Build history of the part. All positions in model axes, mm. A direction names the side the tool comes from. Round coordinates to 2 decimals unless told otherwise and drop trailing zeros. Loops run counter-clockwise (first coordinate to the right, second up) from the corner with the lowest first, then second, coordinate; pieces in that order, holes last.
Autodesk Inventor part; units mm, degrees
ref_plane "YZ Plane" through (0, 0, 0) normal (1, 0, 0) x (0, 1, 0)
ref_plane "XZ Plane" through (0, 0, 0) normal (0, 1, 0) x (-1, 0, 0)
ref_plane "XY Plane" through (0, 0, 0) normal (0, 0, 1) x (1, 0, 0)
sketch "スケッチ1" plane through (0, 0, 0) normal (0, 0, 1) x (1, 0, 0)
  line L0 (0, -3.25) -> (0.8, -3.25)
  line L1 (0.8, -3.25) -> (1.1, -2.95)
  line L2 (1.1, -2.95) -> (1.1, 1.25)
  line L3 (1.1, 1.25) -> (1.1, 1.25)
  line L4 (1.1, 1.25) -> (1.1, 1.75)
  line L5 (1.1, 1.75) -> (2.2, 1.75)
  line L6 (2.5, 5.45) -> (2.2, 5.75)
  line L7 (2.2, 5.75) -> (1.5, 5.75)
  line L8 (1.5, 5.75) -> (1.2, 5.45)
  line L9 (0, 7.4044) -> (0, -7.4044) construction
  line L10 (0, -3.25) -> (0, 3.25)
  line L11 (0, 3.25) -> (1.2, 3.25)
  line L12 (1.2, 3.25) -> (1.2, 5.45)
  line L13 (2.2, 1.75) -> (2.5, 2.05)
  line L14 (2.5, 2.05) -> (2.5, 5.45)
  point P0 (0, 0)
  point P1 (0, 0)
  dimension "d0" = 2.2
  dimension "d1" = 5
  dimension "d2" = 0.3
  dimension "d3" = 0.3
  dimension "d4" = 2.2
  dimension "d5" = 0.5
  dimension "d6" = 4
  dimension "d8" = 0.3
  dimension "d9" = 2.4
  dimension "d10" = 2.5
  dimension "d11" = 0.3
  dimension "d12" = 0.3
  dimension "d13" = 0.3
  dimension "d14" = 0.3
  dimension "d15" = 5
revolve "回転1" add sketch "スケッチ1" angle 360 about axis through (0, 7.4044, 0) along (0, -1, 0)
sketch "スケッチ2" plane through (0, -3.25, 0) normal (0, -1, 0) x (1, 0, 0)
  circle A0 centre (0, 0) radius 0.8
  circle A1 centre (0, 0) radius 9.0242
extrude "押し出し1" cut sketch "スケッチ2" against normal blind 0.5 contours A0 | A1
sketch "スケッチ3" plane through (0, 5.75, 0) normal (0, 1, 0) x (1, 0, 0)
  circle A0 centre (0, 0) radius 2.5
  line L0 (2.5, 0) -> (-2.5, 0)
  line L1 (2.5, -0.5) -> (-2.5, -0.5)
  line L2 (2.5, 0.5) -> (-2.5, 0.5)
  line L3 (2.5, -0.5) -> (2.5, 0.5)
  line L4 (-2.5, -0.5) -> (-2.5, 0.5)
  point P0 (0, 0)
  point P1 (-2.4495, -0.5)
  point P2 (2.4495, -0.5)
  point P3 (2.4495, 0.5)
  point P4 (-2.4495, 0.5)
  dimension "d19" = 0.5
extrude "押し出し2" cut sketch "スケッチ3" against normal blind 1 contours L0 A0 L2 | A0 L1 L0
equation "\"d3\" = d2"
equation "\"d11\" = d8"
equation "\"d12\" = d8"
equation "\"d13\" = d12"
equation "\"d14\" = d13"
properties part number "BRU-2604S" material "ステンレス鋼 AISI 304"
(1) Pull direction X, two halves, no side cores. Call faces 6 (the face through (1.05, -0.47, -0.33)), 7 (the face through (-0.02, 5.57, 1.32)), 8 (the face through (2, 5, -0.5)): +X half, -X half, draft (parallel to the pull), parting line (faces both ways), or undercut.
Responses:
face 6: parting line
face 7: undercut
face 8: draft
(2) Slice it at B-B on x = 0. List the corners of the cut face in (y, z).
Responses:
outline: (-2.75, -1.1) - (1.75, -1.1) - (1.75, -2.2) - (2.05, -2.5) - (5.45, -2.5) - (5.75, -2.2) - (5.75, -1.5) - (5.45, -1.2) - (3.25, -1.2) - (3.25, 1.2) - (5.45, 1.2) - (5.75, 1.5) - (5.75, 2.2) - (5.45, 2.5) - (2.05, 2.5) - (1.75, 2.2) - (1.75, 1.1) - (-2.75, 1.1) - close
(3) Slice it at D-D on y = 4. List the corners of the cut face in (x, z).
Responses:
outline: circle Ø5 at (0, 0); hole circle Ø2.4 at (0, 0)
(4) Slice it at C-C on y = -1.5. List the corners of the cut face in (x, z), plus the area to 3 significant figures.
Responses:
outline: circle Ø2.2 at (0, 0)
area: 3.80 mm2
(5) Slice it at A-A on z = 0. List the corners of the cut face in (x, y).
Responses:
outline: (-2.5, 2.05) - (-2.2, 1.75) - (-1.1, 1.75) - (-1.1, -2.75) - (1.1, -2.75) - (1.1, 1.75) - (2.2, 1.75) - (2.5, 2.05) - (2.5, 4.75) - (1.2, 4.75) - (1.2, 3.25) - (-1.2, 3.25) - (-1.2, 4.75) - (-2.5, 4.75) - close
(6) Which spindle directions (+Z, -Z, +X, -X, +Y, -Y) get a long thin tool onto all of the face, cutting with end or side? Do faces 1 (the face through (0, 5.75, 2)), 2 (the face through (-2, 5, -0.5)), 3 (the face through (2.385, 3.774, -0.751)), 4 (the face through (-1, 1.75, 1)), 5 (the face through (-1.2, 4.37, -0.05)). Say none if no direction does.
Responses:
face 1: +Z, -Z, +X, -X, +Y
face 2: +X, -X, +Y
face 3: +Y, -Y
face 4: -Y
face 5: +Y
(7) Probe line 1 (Z direction, x = 0, y = 4.7); line 2 (X direction, y = 4.25, z = -0.8). List the from-to ranges inside material, lowest first.
Responses:
line 1: z = -2.5 to -1.2, 1.2 to 2.5
line 2: x = -2.37 to -0.89, 0.89 to 2.37
(8) Pin check, flat tips, straight feed: P1, Ø0.5, axis at x = 2, z = 0, coming from the +Y side; P2, Ø0.5, axis at x = -2, y = 5.5, coming from the +Z side; P3, Ø1.5, axis at x = -1.5, y = 0.5, coming from the -Z side. Stop position of each tip, or through.
Responses:
P1: stops at y = 4.75
P2: stops at z = 1.78
P3: stops at z = -0.8
